Study the drawing (mm; zero at the part's minimum x, y, z) and answer. A direction names the side the tool comes from. Coordinates: 2 decimals unless noted, no trailing zeros. Order: outer loops, then holes, each group sorted by start corner. A loop starts at its lowest first (then second) coordinate and runs counter-clockwise, first axis right, second up. Notation, with made-up numbers: (59.25, 62) -> (110.25, 62) arc R20 cw to (110.25, 99) -> close; hole circle Ø6 at (-20.75, 85). An arc over 180 degrees is marked (long way). Answer as CSV lines item,"result". Start each with the question number.
Item 1: Section C-C (x = 34) is taken. Write down the section's boundary in (y, z), then the cut area to 3 significant figures.
Item 2: Section A-A (z = 4.2) is taken. Count the separate pieces of the cut face and the enclosed holes in it, then the cut area to 3 significant figures.
Item 3: Section B-B (x = 29.5) is taken. Write down the section's boundary in (y, z).
Item 4: Which of the six approach directions +Z, -Z, +X, -X, +Y, -Y give full straight-line access (tool end or side, diameter ignored) to the marked faces 4, 5 and 6?
Item 5: For a pull along X with two mould halves and no side action, classify the marked faces 1, 2 and 3 as pulls with the +X half, pulls with the -X half, needs draft (parallel to the pull), parting line crosses it, or undercut.
Item 6: Straight lines are drawn through the part: L1, parallel to X at y = 4, z = 3.7; L2, parallel to Y at x = 34.5, z = 3.6; L3, parallel to Y at x = 19, z = 3.55. For each, find the intervals that lie inside material, in ascending order.
Item 7: Each of these flat-tipped pins is pushed along its axis until it touches: pin 1 Ø3 at (x, y) = (3, 3) entering from -Z; pin 2 Ø10 at (x, y) = (17.5, 22) entering from +Z; pin 3 Ø1.6 at (y, z) = (24, 1) entering from +X. Where does it stop, or does it pass through?
Item 8: Section D-D (y = 10.5) is taken. Write down the section's boundary in (x, z).
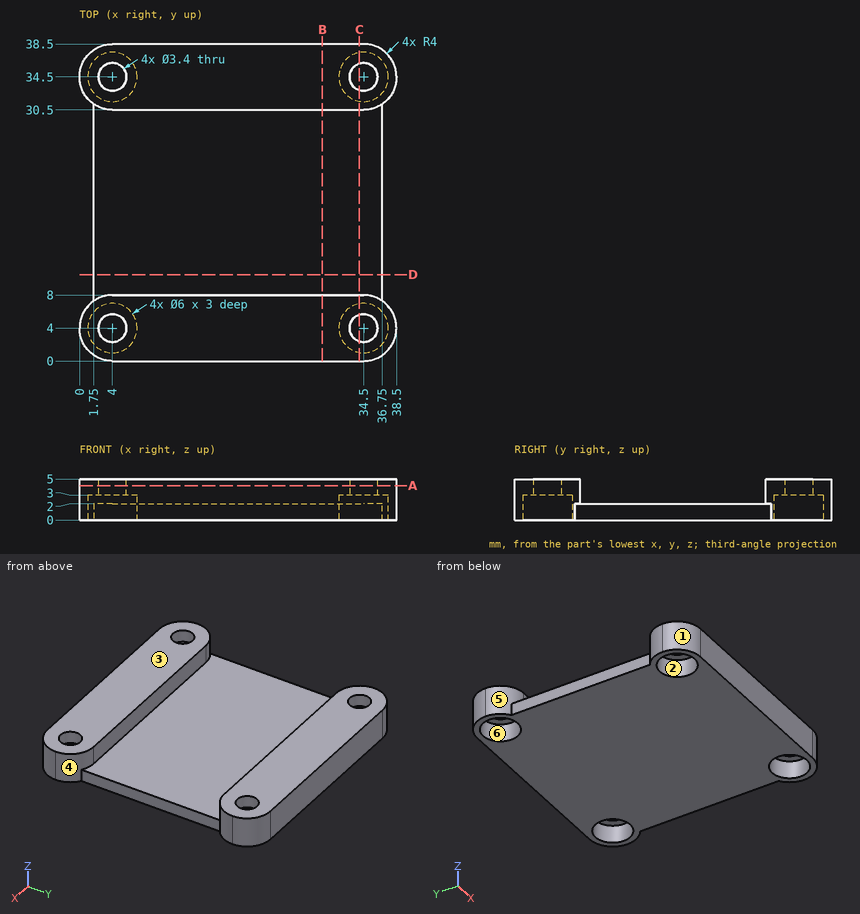
Checked values:
1,outline,"(0, 0) -> (1.04, 0) -> (1.04, 3) -> (2.38, 3) -> (2.38, 5) -> (0, 5) -> close; (5.62, 3) -> (6.96, 3) -> (6.96, 0) -> (31.54, 0) -> (31.54, 3) -> (32.88, 3) -> (32.88, 5) -> (30.5, 5) -> (30.5, 2) -> (8, 2) -> (8, 5) -> (5.62, 5) -> close; (36.12, 3) -> (37.46, 3) -> (37.46, 0) -> (38.5, 0) -> (38.5, 5) -> (36.12, 5) -> close"
1,area,"76.5 mm^2"
2,separate pieces,"2"
2,enclosed holes,"4"
2,area,"552 mm^2"
3,outline,"(0, 0) -> (38.5, 0) -> (38.5, 5) -> (30.5, 5) -> (30.5, 2) -> (8, 2) -> (8, 5) -> (0, 5) -> close"
4,face 4,"+Z, +X"
4,face 5,"+Z, -X"
4,face 6,"-Z"
5,face 1,"pulls with the -X half"
5,face 2,"undercut"
5,face 3,"needs draft"
6,L1,"x = 0 to 2.3, 5.7 to 32.8, 36.2 to 38.5"
6,L2,"y = 0 to 2.3, 5.7 to 8, 30.5 to 32.8, 36.2 to 38.5"
6,L3,"y = 0 to 8, 30.5 to 38.5"
7,pin 1,"stops at z = 3"
7,pin 2,"stops at z = 2"
7,pin 3,"stops at x = 36.75"
8,outline,"(1.75, 0) -> (36.75, 0) -> (36.75, 2) -> (1.75, 2) -> close"
